```python
from build123d import *

# Parameters (mm, degrees)
SKETCH1_R                       = 4
BOSS_EXTRUDE1_DEPTH             = 200
SKETCH2_R                       = 11
BOSS_EXTRUDE2_DEPTH             = 2
SKETCH3_W                       = 42.418
SKETCH3_H                       = 42.418
BOSS_EXTRUDE3_DEPTH             = 48
CUT_EXTRUDE1_DEPTH              = 250.80721239
M3X0_5_TAPPED_HOLE1_D           = 2.5
M3X0_5_TAPPED_HOLE1_DEPTH       = 7.5
M3X0_5_TAPPED_HOLE1_CBORE_D     = 3
M3X0_5_TAPPED_HOLE1_CBORE_DEPTH = 6
M3X0_5_TAPPED_HOLE1_TIP         = 0.751075774
CUT_EXTRUDE3_DEPTH              = 15.25


with BuildPart() as part:
    # Sketch1 → Boss-Extrude1 (new body)
    with BuildSketch(Plane.XY):
        Circle(SKETCH1_R)
    extrude(amount=BOSS_EXTRUDE1_DEPTH)

    # Sketch2 → Boss-Extrude2 (add)
    with BuildSketch(Plane(origin=(0, 0, 0), x_dir=(-1, 0, 0), z_dir=(0, 0, -1))):
        Circle(SKETCH2_R)
    extrude(amount=-BOSS_EXTRUDE2_DEPTH)

    # Sketch3 → Boss-Extrude3 (add)
    with BuildSketch(Plane(origin=(0, 0, 0), x_dir=(-1, 0, 0), z_dir=(0, 0, -1))):
        Rectangle(SKETCH3_W, SKETCH3_H)
    extrude(amount=BOSS_EXTRUDE3_DEPTH)

    # Sketch4 → Cut-Extrude1 (cut, through all)
    with BuildSketch(Plane(origin=(0, 0, -48), x_dir=(-1, 0, 0), z_dir=(0, 0, -1))):
        with BuildLine():
            Line((-21.209, -15.887992919), (-21.209, -21.209))
            Line((-21.209, -21.209), (-15.887992919, -21.209))
            ThreePointArc((-15.887992919, -21.209), (-18.738329701, -18.738329701), (-21.209, -15.887992919))
        make_face()
        with BuildLine():
            Line((15.887992919, -21.209), (21.209, -21.209))
            Line((21.209, -21.209), (21.209, -15.887992919))
            ThreePointArc((21.209, -15.887992919), (18.738329701, -18.738329701), (15.887992919, -21.209))
        make_face()
        with BuildLine():
            Line((21.209, 15.887992919), (21.209, 21.209))
            Line((21.209, 21.209), (15.887992919, 21.209))
            ThreePointArc((15.887992919, 21.209), (18.738329701, 18.738329701), (21.209, 15.887992919))
        make_face()
        with BuildLine():
            Line((-15.887992919, 21.209), (-21.209, 21.209))
            Line((-21.209, 21.209), (-21.209, 15.887992919))
            ThreePointArc((-21.209, 15.887992919), (-18.738329701, 18.738329701), (-15.887992919, 21.209))
        make_face()
    extrude(amount=-CUT_EXTRUDE1_DEPTH, mode=Mode.SUBTRACT)

    # M3x0.5 Tapped Hole1
    with Locations(Plane.XY):
        with Locations((-15.5, 15.5), (-15.5, -15.5), (15.5, -15.5), (15.5, 15.5)):
            CounterBoreHole(M3X0_5_TAPPED_HOLE1_D / 2, M3X0_5_TAPPED_HOLE1_CBORE_D / 2, M3X0_5_TAPPED_HOLE1_CBORE_DEPTH, depth=M3X0_5_TAPPED_HOLE1_DEPTH)
            with Locations((0, 0, -(M3X0_5_TAPPED_HOLE1_DEPTH + M3X0_5_TAPPED_HOLE1_TIP / 2))):  # 118° drill point
                Cone(0, M3X0_5_TAPPED_HOLE1_D / 2, M3X0_5_TAPPED_HOLE1_TIP, mode=Mode.SUBTRACT)

    # Sketch8 → Cut-Extrude3 (cut, symmetric)
    with BuildSketch(Plane.XY.offset(-24)):
        with BuildLine():
            Line((15.887992919, 21.209), (-15.887992919, 21.209))
            ThreePointArc((-15.887992919, 21.209), (-18.738329701, 18.738329701), (-21.209, 15.887992919))
            Line((-21.209, 15.887992919), (-21.209, -15.887992919))
            ThreePointArc((-21.209, -15.887992919), (-18.738329701, -18.738329701), (-15.887992919, -21.209))
            Line((-15.887992919, -21.209), (15.887992919, -21.209))
            ThreePointArc((15.887992919, -21.209), (18.738329701, -18.738329701), (21.209, -15.887992919))
            Line((21.209, -15.887992919), (21.209, 15.887992919))
            ThreePointArc((21.209, 15.887992919), (18.738329701, 18.738329701), (15.887992919, 21.209))
        make_face()
        with BuildLine():
            Line((-13.394406258, 21.109), (13.394406258, 21.109))
            ThreePointArc((13.394406258, 21.109), (17.67766953, 17.67766953), (21.109, 13.394406258))
            Line((21.109, 13.394406258), (21.109, -13.394406258))
            ThreePointArc((21.109, -13.394406258), (17.67766953, -17.67766953), (13.394406258, -21.109))
            Line((13.394406258, -21.109), (-13.394406258, -21.109))
            ThreePointArc((-13.394406258, -21.109), (-17.67766953, -17.67766953), (-21.109, -13.394406258))
            Line((-21.109, -13.394406258), (-21.109, 13.394406258))
            ThreePointArc((-21.109, 13.394406258), (-17.67766953, 17.67766953), (-13.394406258, 21.109))
        make_face(mode=Mode.SUBTRACT)
    extrude(amount=CUT_EXTRUDE3_DEPTH, both=True, mode=Mode.SUBTRACT)


solid = part.part
```
Could you check a few things on this model? Use its own coordinates, in mm. A direction names the side the tool comes from. Give positions to 0.01 mm unless a question says otherwise; leave off trailing zeros. Write each loop counter-clockwise with the first axis right and the second up, starting at its lowest first coordinate (ties: lowest second). Pieces come first, ordered by that corner, then holes. Notation, with made-up numbers: (62.5, 63) - (111.5, 63) arc R28 ccw to (111.5, 100) - close; hole circle Ø4 at (87, 3.25). An arc over 180 degrees is marked (long way). One line per item, written item: value. Start each with the question number.
Item 1: I'm going to push flat-ended pins straight in: pin 1 (3.5 mm diameter, centred on x = 15.5, y = -15.5, fed in from +Z); pin 2 (1.8 mm diameter, centred on x = -15.5, y = -15.5, fed in from +Z); pin 3 (6 mm diameter, centred on y = -3, z = 41.5, fed in from -X). Where does each tip first touch, or does it pass through?
Item 2: If we mould it in two halves opening along Z, with no side actions, what happens to faces 4 (the face through (18.701, -18.776, -43.686)), 5 (the face through (0, 0, -48)), 6 (the face through (17.732, -17.623, -23.786))? For each: +Z half, -Z half, draft (parallel to the pull), parting line (faces both ways), or undercut.
Item 3: Which directions (+Z, -Z, +X, -X, +Y, -Y) give clear straight access to the entire face, cutting with the end or side of a thin tool? Please do faces 1 (the face through (-17.732, 17.623, -23.786)), 2 (the face through (-17.623, -17.732, -23.786)), 3 (the face through (0, -5, 2)).
Item 4: Please list where these lines run through material, in increasing order: line 1 (Y direction, x = -15.5, z = -2.7); line 2 (Y direction, x = 15.5, z = -6.9). Write a range as from..to.
Item 5: Imagine slicing it at B-B, the plane z = 61.5. List the corners of the cut face in (x, y) for me.
Item 6: Imagine slicing it at A-A, the plane x = 0. List the corners of the cut face in (y, z) for me, and give its area (3 significant figures).
Geometry says:
1. pin 1: z = 0
1. pin 2: z = -7.71
1. pin 3: x = -4
2. face 4: draft
2. face 5: -Z half
2. face 6: undercut
3. face 1: -X, +Y
3. face 2: -X, -Y
3. face 3: +Z
4. line 1: -21.21..-17, -14..14, 17..21.21
4. line 2: -21.21..-16.75, -14.25..14.25, 16.75..21.21
5. outline: circle Ø8 at (0, 0)
6. outline: (-21.21, -48) - (21.21, -48) - (21.21, -39.25) - (21.11, -39.25) - (21.11, -8.75) - (21.21, -8.75) - (21.21, 0) - (11, 0) - (11, 2) - (4, 2) - (4, 200) - (-4, 200) - (-4, 2) - (-11, 2) - (-11, 0) - (-21.21, 0) - (-21.21, -8.75) - (-21.11, -8.75) - (-21.11, -39.25) - (-21.21, -39.25) - close
6. area: 3,660 mm^2
